from build123d import *

# Parameters (mm, degrees)
SKETCH1_R                = 0.5
BOSS_EXTRUDE1_DEPTH      = 1.15
BOSS_EXTRUDE2_DEPTH      = 1
BOSS_EXTRUDE2_DEPTH_BACK = 3.6
SKETCH2_R                = 0.25
SKETCH3_W                = 2.5
SKETCH3_H                = 5
BOSS_EXTRUDE3_DEPTH      = 4.7
CUT_EXTRUDE1_DEPTH       = 0.05
FILLET1_R                = 0.9


with BuildPart() as part:
    # Sketch1 → Boss-Extrude1 (new body)
    with BuildSketch(Plane(origin=(0, 0, 0), x_dir=(1, 0, 0), z_dir=(0, 1, 0))):
        Polygon((0, 0), (0, 16.5), (4.45, 16.5), (4.45, 10), (6.55, 10), (6.55, 16.5), (11, 16.5), (11, 0), align=None)
        with Locations(Location((9.5, 1.5, 0), (0, 0, 270))):
            Circle(SKETCH1_R, mode=Mode.SUBTRACT)
        with Locations(Location((7.833333333, 1.5, 0), (0, 0, 270))):
            Circle(SKETCH1_R, mode=Mode.SUBTRACT)
        with Locations(Location((6.166666667, 1.5, 0), (0, 0, 270))):
            Circle(SKETCH1_R, mode=Mode.SUBTRACT)
        with Locations(Location((4.5, 1.5, 0), (0, 0, 270))):
            Circle(SKETCH1_R, mode=Mode.SUBTRACT)
    extrude(amount=BOSS_EXTRUDE1_DEPTH)

    # Sketch2 → Boss-Extrude2 (add, two sides: drawn at the far end of the back side and taken through both)
    with BuildSketch(Plane(origin=(0, 1.15, 0), x_dir=(1, 0, 0), z_dir=(0, 1, 0)).offset(-BOSS_EXTRUDE2_DEPTH_BACK)):
        with Locations(Location((2.303324378, 14.15500421, 0), (0, 0, 270))):
            Circle(SKETCH2_R)
        with Locations(Location((2.303324378, 11.151722015, 0), (0, 0, 270))):
            Circle(SKETCH2_R)
        with Locations(Location((8.916612443, 11.151722015, 0), (0, 0, 270))):
            Circle(SKETCH2_R)
        with Locations(Location((8.916612443, 14.15500421, 0), (0, 0, 270))):
            Circle(SKETCH2_R)
    extrude(amount=BOSS_EXTRUDE2_DEPTH + BOSS_EXTRUDE2_DEPTH_BACK)

    # Sketch3 → Boss-Extrude3 (add)
    with BuildSketch(Plane.XZ.offset(2.45)):
        with Locations((2.303324378, -12.637884748)):
            Rectangle(SKETCH3_W, SKETCH3_H)
        with Locations((8.916612443, -12.637884748)):
            Rectangle(SKETCH3_W, SKETCH3_H)
    extrude(amount=BOSS_EXTRUDE3_DEPTH)

    # Sketch4 → Cut-Extrude1 (cut)
    with BuildSketch(Plane(origin=(0, 1.15, 0), x_dir=(1, 0, 0), z_dir=(0, 1, 0))):
        with BuildLine():
            Line((3.901788048, 1), (3.901788048, 2))
            ThreePointArc((3.901788048, 2), (4.5, 2.598211952), (5.098211952, 2))
            Line((5.098211952, 2), (5.098211952, 1))
            ThreePointArc((5.098211952, 1), (4.5, 0.401788048), (3.901788048, 1))
        make_face()
        with BuildLine():
            Line((5.568454715, 1), (5.568454715, 2))
            ThreePointArc((5.568454715, 2), (6.166666667, 2.598211952), (6.764878619, 2))
            Line((6.764878619, 2), (6.764878619, 1))
            ThreePointArc((6.764878619, 1), (6.166666667, 0.401788048), (5.568454715, 1))
        make_face()
        with BuildLine():
            Line((7.235121381, 1), (7.235121381, 2))
            ThreePointArc((7.235121381, 2), (7.833333333, 2.598211952), (8.431545285, 2))
            Line((8.431545285, 2), (8.431545285, 1))
            ThreePointArc((8.431545285, 1), (7.833333333, 0.401788048), (7.235121381, 1))
        make_face()
        with BuildLine():
            Line((8.901788048, 1), (8.901788048, 2))
            ThreePointArc((8.901788048, 2), (9.5, 2.598211952), (10.098211952, 2))
            Line((10.098211952, 2), (10.098211952, 1))
            ThreePointArc((10.098211952, 1), (9.5, 0.401788048), (8.901788048, 1))
        make_face()
    extrude(amount=-CUT_EXTRUDE1_DEPTH, mode=Mode.SUBTRACT)

    # Fillet1
    fillet1_edges = [part.edges().sort_by_distance(p)[0] for p in [
        (2.303324378, 1.15, -14.40500421),
        (2.303324378, 1.15, -11.401722015),
        (8.916612443, 1.15, -11.401722015),
        (8.916612443, 1.15, -14.40500421),
    ]]
    fillet(fillet1_edges, radius=FILLET1_R)


solid = part.part
Input: part model. Units: mm. Frame: model coordinates. A direction names the side the tool comes from. Round coordinates to 2 decimals unless told otherwise and drop trailing zeros. Order: outer loops, then holes, each group sorted by start corner. A loop starts at its lowest first (then second) coordinate and runs counter-clockwise, first axis right, second up.
1. Cut plane C-C, the plane z = -1.5. State how many separate pieces and enclosed holes the cut face has, then the cut area to 3 significant figures.
The answers:
separate pieces: 5
enclosed holes: 0
area: 8.01 mm2
2. Mould query, pull axis Z, two halves, no side actions, for faces 1 (the face through (9, -5, -15.138)), 2 (the face through (9, -7.15, -13)), 3 (the face through (4.996, 0.542, -1.565)). Classes: released by +Z, released by -Z, zero draft, split by the parting line, or undercut.
The answers:
face 1: released by -Z
face 2: zero draft
face 3: undercut
3. Cut plane B-B, the plane z = -12.5. Output: boundary loops of the cut face in (x, y).
The answers:
outline: (0, 0) - (4.45, 0) - (4.45, 1.15) - (0, 1.15) - close; (1.05, -7.15) - (3.55, -7.15) - (3.55, -2.45) - (1.05, -2.45) - close; (6.55, 0) - (11, 0) - (11, 1.15) - (6.55, 1.15) - close; (7.67, -7.15) - (10.17, -7.15) - (10.17, -2.45) - (7.67, -2.45) - close
4. Set-up query: faces 4 (the face through (6.55, 0.6, -13.2)), 5 (the face through (7.667, -5, -13)), 6 (the face through (1.053, -5, -13)), 7 (the face through (2, -5, -10.138)). Return all of +Z, -Z, +X, -X, +Y, -Y with unobstructed straight access to the full face (end or side cutting, diameter ignored); none if empty.
The answers:
face 4: -Z, +Y, -Y
face 5: +Z, -Z, -Y
face 6: +Z, -Z, -X, -Y
face 7: +Z, +X, -X, -Y
5. Pin query (flat end, axial travel): P1, Ø0.8, axis at x = 2, y = -6, coming from the +Z side; P2, Ø2, axis at x = 2.5, z = -5.5, coming from the -Y side; P3, Ø5, axis at y = -4, z = -12.5, coming from the -X side. Return the tip coordinate at first contact, or that it passes through.
The answers:
P1: stops at z = -10.14
P2: stops at y = 0
P3: stops at x = 1.05
6. Cut plane A-A, the plane y = -5.25. Output: boundary loops of the cut face in (x, z), then the cut area to 3 significant figures.
The answers:
outline: (1.05, -15.14) - (3.55, -15.14) - (3.55, -10.14) - (1.05, -10.14) - close; (7.67, -15.14) - (10.17, -15.14) - (10.17, -10.14) - (7.67, -10.14) - close
area: 25.0 mm2
7. Material intervals for line 1 (X direction, y = 0.35, z = -1.5); line 2 (X direction, y = -5.75, z = -13.5); line 3 (Y direction, x = 4, z = -12.25), sorted ascending.
The answers:
line 1: x = 0 to 4, 5 to 5.67, 6.67 to 7.33, 8.33 to 9, 10 to 11
line 2: x = 1.05 to 3.55, 7.67 to 10.17
line 3: y = 0 to 1.15
